Model file for the job. Use its own axes, mm. Face numbers are marked on the shaded views. Round coordinates to 2 decimals unless told otherwise and drop trailing zeros. Order: outer loops, then holes, each group sorted by start corner. A loop starts at its lowest first (then second) coordinate and runs counter-clockwise, first axis right, second up. Notation, with made-up numbers: (-38.5, 67.25) - (0.5, 67.25) arc R23 ccw to (0.5, 85.25) - close; hole circle Ø8 at (65, 37.5). An arc over 180 degrees is marked (long way). Use one line per item in the form item = value.
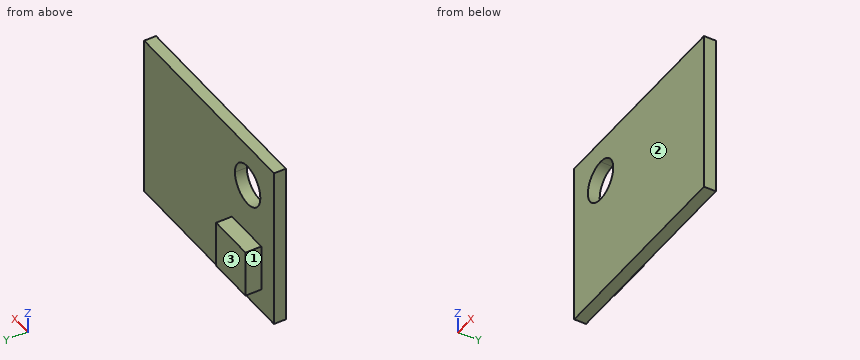
from build123d import *

# Parameters (mm, degrees)
F1_DEPTH = 0.375
F2_W     = 3
F2_H     = 3
F3_DEPTH = 1


with BuildPart() as f1:
    # F0 (on Front) → F1 (new body, symmetric)
    with BuildSketch(Plane.XZ):
        Polygon((6.65, -5.25), (6.65, 5.25), (-3.95, 5.25), (-6.65, 5.25), (-6.65, -5.25), align=None)
        with BuildLine():
            ThreePointArc((-2.65, 2.55), (-4.869239, 1.630761), (-3.95, 3.85))
            ThreePointArc((-3.95, 3.85), (-3.030761, 3.469239), (-2.65, 2.55))
        make_face(mode=Mode.SUBTRACT)
    extrude(amount=F1_DEPTH, both=True)

    # F2 (on face) → F3 (join)
    with BuildSketch(Plane(origin=(0, 0.375, 0), x_dir=(-1, 0, 0), z_dir=(0, 1, 0))):
        with Locations((3.85, -2.25)):
            Rectangle(F2_W, F2_H)
    extrude(amount=F3_DEPTH)


solid = f1.part
(1) Slice it at B-B on x = -3.75. Give the cut face in (y, z) (3 decimals), then the cut area to 3 significant figures.
Report:
outline = (-0.375, -5.25) - (0.375, -5.25) - (0.375, -3.75) - (1.375, -3.75) - (1.375, -0.75) - (0.375, -0.75) - (0.375, 1.265) - (-0.375, 1.265) - close; (-0.375, 3.835) - (0.375, 3.835) - (0.375, 5.25) - (-0.375, 5.25) - close
area = 8.95 mm2
(2) Slice it at D-D on y = 0.9. Give the cut face in (x, z).
Report:
outline = (-5.35, -3.75) - (-2.35, -3.75) - (-2.35, -0.75) - (-5.35, -0.75) - close
(3) Probe probe 1 along Z at (x, y) = (-3.95, 0.15); probe 2 along Z at (x, y) = (-4, 0.95); probe 3 along Y at (x, z) = (1, 3) (3 decimals). List the from-to ranges inside material, lowest first. Write a range as [from, to].
Report:
probe_1 = [-5.25, 1.25], [3.85, 5.25]
probe_2 = [-3.75, -0.75]
probe_3 = [-0.375, 0.375]
(4) Pull direction Y, two halves, no side cores. Call the marked faces 1, 2 and 3: released by +Y, released by -Y, zero draft, split by the parting line, or undercut.
Report:
face_1 = zero draft
face_2 = released by -Y
face_3 = released by +Y
(5) Pin check, flat tips, straight feed: pin 1 (5 mm diameter, centred on x = 1, z = -3.5, fed in from +Y) (3 decimals); pin 2 (0.5 mm diameter, centred on x = -4.5, y = 1, fed in from +Z). Stop position of each tip, or through.
Report:
pin_1 = 0.375
pin_2 = -0.75
(6) Slice it at C-C on z = -1.5. Give the cut face in (x, y) (3 decimals).
Report:
outline = (-6.65, -0.375) - (6.65, -0.375) - (6.65, 0.375) - (-2.35, 0.375) - (-2.35, 1.375) - (-5.35, 1.375) - (-5.35, 0.375) - (-6.65, 0.375) - close
(7) Slice it at A-A on z = 2.25. Give the cut face in (x, y) (3 decimals).
Report:
outline = (-6.65, -0.375) - (-5.215, -0.375) - (-5.215, 0.375) - (-6.65, 0.375) - close; (-2.685, -0.375) - (6.65, -0.375) - (6.65, 0.375) - (-2.685, 0.375) - close
